from build123d import *

# Parameters (mm, degrees)
CROQUIS1_R              = 4
SALIENTE_EXTRUIR1_DEPTH = 2
CROQUIS3_W              = 6.205121333
CROQUIS3_H              = 2
SALIENTE_EXTRUIR2_DEPTH = 24.5
CROQUIS4_W              = 6.205121333
CROQUIS4_H              = 2
SALIENTE_EXTRUIR3_DEPTH = 8


with BuildPart() as part:
    # Croquis1 → Saliente-Extruir1 (new body)
    with BuildSketch(Plane.XY):
        with BuildLine():
            Line((-3.36280679, 16.435636067), (-3.36280679, 7.2588932))
            ThreePointArc((-3.36280679, 7.2588932), (0.282374909, -7.995014973), (2.842314543, 7.478051086))
            Line((2.842314543, 7.478051086), (2.842314543, 16.435636067))
            Line((2.842314543, 16.435636067), (-3.36280679, 16.435636067))
        make_face()
        Circle(CROQUIS1_R, mode=Mode.SUBTRACT)
    extrude(amount=SALIENTE_EXTRUIR1_DEPTH)

    # Croquis3 → Saliente-Extruir2 (add)
    with BuildSketch(Plane(origin=(0, 16.435636067, 0), x_dir=(1, 0, 0), z_dir=(0, 1, 0))):
        with Locations((-0.260246123, -1)):
            Rectangle(CROQUIS3_W, CROQUIS3_H)
    extrude(amount=SALIENTE_EXTRUIR2_DEPTH)

    # Croquis4 → Saliente-Extruir3 (add)
    with BuildSketch(Plane(origin=(0, 40.935636067, 0), x_dir=(1, 0, 0), z_dir=(0, 1, 0))):
        with Locations((-0.260246123, -1)):
            Rectangle(CROQUIS4_W, CROQUIS4_H)
    extrude(amount=SALIENTE_EXTRUIR3_DEPTH)


solid = part.part
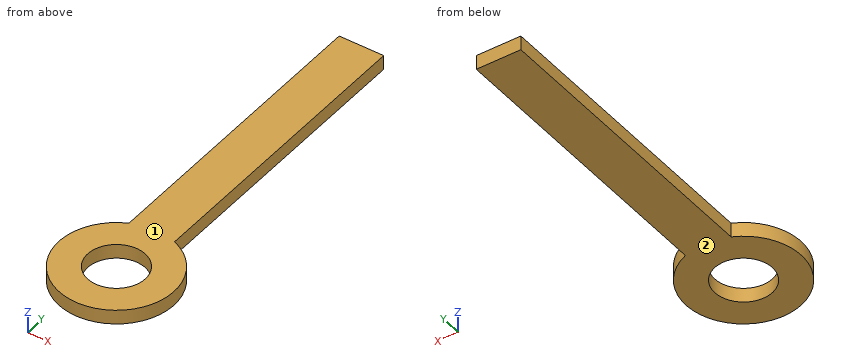
Check sheet for the modelled part. Datum: model origin and axes. Units: mm. Face numbers are marked on the shaded views. Coordinates: 2 decimals unless noted, no trailing zeros. Write each loop counter-clockwise with the first axis right and the second up, starting at its lowest first coordinate (ties: lowest second). Pieces come first, ordered by that corner, then holes.
Item 1: Mould release check, pull along Z, two halves, no side actions. Record for the marked faces 1 and 2: released by +Z, released by -Z, zero draft, split by the parting line, or undercut.
Numbers:
face 1: released by +Z
face 2: released by -Z
Item 2: Cross-section at D-D on y = 21. Record the boundary of the cut face in (x, z), then the cut area to 3 significant figures.
Numbers:
outline: (-3.36, 0) - (2.84, 0) - (2.84, 2) - (-3.36, 2) - close
area: 12.4 mm2
Item 3: Cross-section at C-C on y = 0. Record the boundary of the cut face in (x, z), then the cut area to 3 significant figures.
Numbers:
outline: (-8, 0) - (-4, 0) - (-4, 2) - (-8, 2) - close; (4, 0) - (8, 0) - (8, 2) - (4, 2) - close
area: 16.0 mm2
Item 4: Scan lines: probe 1 along Y at (x, z) = (0, 0.7); probe 2 along X at (y, z) = (8, 0.15); probe 3 along Y at (x, z) = (-2.5, 1.3). Record each from-to range of solid material in increasing order.
Numbers:
probe 1: y = -8 to -4, 4 to 48.94
probe 2: x = -3.36 to 2.84
probe 3: y = -7.6 to -3.12, 3.12 to 48.94
Item 5: Cross-section at B-B on z = 1.05. Record the boundary of the cut face in (x, y).
Numbers:
outline: (-3.36, 7.26) arc R8 ccw (long way) to (2.84, 7.48) - (2.84, 48.94) - (-3.36, 48.94) - close; hole circle Ø8 at (0, 0)
Item 6: Cross-section at A-A on x = 0. Record the boundary of the cut face in (y, z).
Numbers:
outline: (-8, 0) - (-4, 0) - (-4, 2) - (-8, 2) - close; (4, 0) - (48.94, 0) - (48.94, 2) - (4, 2) - close
